from build123d import *

# Parameters (mm, degrees)
F0_R     = 1.5
F1_DEPTH = 10


with BuildPart() as f1:
    # F0 (on Top) → F1 (new body)
    with BuildSketch(Plane.XY):
        with BuildLine():
            ThreePointArc((13, 2.526602), (7.800135, 1.906809), (3, 4))
            ThreePointArc((3, 4), (-2.236068, 4.472136), (-5, 0))
            ThreePointArc((-5, 0), (-4.993207, -0.260536), (-4.972848, -0.520364))
            ThreePointArc((-4.972848, -0.520364), (-5.4, -7.2), (0.892848, -4.919636))
            ThreePointArc((0.892848, -4.919636), (2, -4.582576), (3, -4))
            ThreePointArc((3, -4), (7.800135, -1.906809), (13, -2.526602))
            Line((13, -2.526602), (13, -0.824336))
            ThreePointArc((13, -0.824336), (7.315028, -0.36781), (2.1, -2.676663))
            ThreePointArc((2.1, -2.676663), (1.545471, -3.030849), (0.933132, -3.271665))
            ThreePointArc((0.933132, -3.271665), (-0.6, -0.8), (-3.402075, -0.020259))
            ThreePointArc((-3.402075, -0.020259), (-3.40212, -0.01013), (-3.402136, 0))
            ThreePointArc((-3.402136, 0), (-1.488295, 3.059331), (2.1, 2.676663))
            ThreePointArc((2.1, 2.676663), (7.315028, 0.36781), (13, 0.824336))
            Line((13, 0.824336), (13, 2.526602))
        make_face()
        with Locations((-3, -4)):
            Circle(F0_R, mode=Mode.SUBTRACT)
    extrude(amount=F1_DEPTH)


solid = f1.part
Can you work these out from the model? Positions are in its coordinate system, mm. A direction names the side the tool comes from. Coordinates: 2 decimals unless noted, no trailing zeros. Write each loop counter-clockwise with the first axis right and the second up, starting at its lowest first coordinate (ties: lowest second). Pieces come first, ordered by that corner, then holes. Notation, with made-up numbers: (-38.75, -35.5) - (-31.75, -35.5) arc R19 cw to (-31.75, -9.5) - close; hole circle Ø6 at (22, -14.75). An arc over 180 degrees is marked (long way). Return JSON: item names as keys, results as strings. Group by question number.
Item 1: If we section it at D-D (x = -3): Write out the boundary of the cut face in (y, z), then the cut area to 3 significant figures.
Item 2: If we section it at C-C (y = 1.25): Write out the boundary of the cut face in (x, z), then the cut area to 3 significant figures.
Item 3: I'm going to push flat-ended pins straight in: pin 1 Ø1.5 at (x, z) = (-1.5, 7.5) entering from +Y; pin 2 Ø4 at (x, z) = (4.5, 4) entering from -Y; pin 3 Ø6 at (x, z) = (3.5, 9) entering from -Y; pin 4 Ø2.5 at (x, y) = (-3, -4) entering from -Z. Where does each tip first touch, or does it pass through?
Item 4: If we section it at B-B (x = -0.5): Write out the boundary of the cut face in (y, z).
Item 5: Please list where these lines run through material, in increasing order: probe 1 along Y at (x, z) = (-3, 3); probe 2 along Y at (x, z) = (9.5, 5.25); probe 3 along Y at (x, z) = (8, 3.25).
Item 6: Which directions (+Z, -Z, +X, -X, +Y, -Y) give clear straight access to the entire face, cutting with the end or side of a thin tool? Please do faces 4 (the face through (7.24, 0.38, 4.93)), 5 (the face through (0, -2, 0)).
Item 7: We'd pull the mould along X, two halves only. Please class faces 1 (the face through (0, -2, 10)), 2 (the face through (-2.166, 4.506, 4.93)), 3 (the face through (1.55, -3.03, 4.93)): pulls with the +X half, pulls with the -X half, needs draft (parallel to the pull), parting line crosses it, or undercut.
Return value:
{
 "1": {"outline": "(-8, 0) - (-5.5, 0) - (-5.5, 10) - (-8, 10) - close; (-2.5, 0) - (0, 0) - (0, 10) - (-2.5, 10) - close; (1.6, 0) - (4, 0) - (4, 10) - (1.6, 10) - close", "area": "74.0 mm^2"},
 "2": {"outline": "(-4.84, 0) - (-3.16, 0) - (-3.16, 10) - (-4.84, 10) - close; (4.44, 0) - (13, 0) - (13, 10) - (4.44, 10) - close", "area": "102 mm^2"},
 "3": {"pin 1": "stops at y = 4.94", "pin 2": "stops at y = -4.33", "pin 3": "stops at y = -5.94", "pin 4": "passes through"},
 "4": {"outline": "(-7.12, 0) - (-0.88, 0) - (-0.88, 10) - (-7.12, 10) - close; (3.37, 0) - (4.97, 0) - (4.97, 10) - (3.37, 10) - close"},
 "5": {"probe 1": "y = -8 to -5.5, -2.5 to 0, 1.6 to 4", "probe 2": "y = -1.8 to -0.21, 0.21 to 1.8", "probe 3": "y = -1.88 to -0.27, 0.27 to 1.88"},
 "6": {"face 4": "+Z, -Z", "face 5": "-Z, +X, -X, +Y, -Y"},
 "7": {"face 1": "needs draft", "face 2": "parting line crosses it", "face 3": "undercut"}
}
